Read the model definition and answer for the solid it produces. Units are mm, in the model's axes. Round coordinates to 2 decimals unless told otherwise and drop trailing zeros. Write each loop counter-clockwise with the first axis right and the second up, starting at its lowest first coordinate (ties: lowest second). Pieces come first, ordered by that corner, then holes. Notation, with made-up numbers: (65.25, -26) - (93.25, -26) arc R21 ccw to (93.25, -9) - close; hole circle Ø3 at (-26, 69.25). An arc over 180 degrees is marked (long way). Use one line per item in the form item = value. Start each with the question number.
1) The part is cut by section A-A, the plane y = 3.25. Give the vertices of the cut face in (x, z).
2) The part is cut by section B-B, the plane z = -79.5. Give the vertices of the cut face in (x, y).
3) Consider line 1 along X through (y, z) = (1.05, -15.5); line 2 along Z through (x, y) = (13, 8); line 3 along Z through (x, y) = (57.75, 0.6). Determine where each line is inside the solid, lowest interval first. Write a range as from..to.
4) The part is cut by section D-D, the plane z = -15.5. Give the vertices of the cut face in (x, y).
5) Each of these flat-tipped pins is pushed along its axis until it touches: pin 1 (2 mm diameter, centred on x = 70, y = 3, fed in from -Z); pin 2 (4 mm diameter, centred on x = 111.75, z = -15.5, fed in from +Y); pin 3 (4.5 mm diameter, centred on y = 5, z = -7, fed in from -X). Where does it stop, or does it pass through?
6) The part is cut by section C-C, the plane x = 57.75. Give the vertices of the cut face in (y, z).
from build123d import *

# Parameters (mm, degrees)
SKETCH1_W                = 116
SKETCH1_H                = 100
BOSS_EXTRUDE1_DEPTH      = 1.65
M3_CLEARANCE_HOLE1_D     = 3.2
M3_CLEARANCE_HOLE1_DEPTH = 20
M3_CLEARANCE_HOLE1_TIP   = 0.96137699
SKETCH6_W                = 52.4
SKETCH6_H                = 11.4
SKETCH6_W_2              = 50
SKETCH6_H_2              = 9
EXTRUDE_THIN1_DEPTH      = 9


with BuildPart() as part:
    # Sketch1 → Boss-Extrude1 (new body)
    with BuildSketch(Plane(origin=(0, 0, 0), x_dir=(1, 0, 0), z_dir=(0, 1, 0))):
        with Locations((58, 50)):
            Rectangle(SKETCH1_W, SKETCH1_H)
    extrude(amount=BOSS_EXTRUDE1_DEPTH)

    # M3 Clearance Hole1
    with Locations(Plane(origin=(0, 1.65, 0), x_dir=(1, 0, 0), z_dir=(0, 1, 0))):
        with Locations((4, 15.5), (111.75, 15.5), (57.75, 79.5)):
            Hole(M3_CLEARANCE_HOLE1_D / 2, depth=M3_CLEARANCE_HOLE1_DEPTH)
            with Locations((0, 0, -(M3_CLEARANCE_HOLE1_DEPTH + M3_CLEARANCE_HOLE1_TIP / 2))):  # 118° drill point
                Cone(0, M3_CLEARANCE_HOLE1_D / 2, M3_CLEARANCE_HOLE1_TIP, mode=Mode.SUBTRACT)

    # Sketch6 → Extrude-Thin1 (add)
    with BuildSketch(Plane(origin=(0, 1.65, 0), x_dir=(1, 0, 0), z_dir=(0, 1, 0))):
        with Locations((29, 7.5)):
            Rectangle(SKETCH6_W, SKETCH6_H)
        with Locations((29, 7.5)):
            Rectangle(SKETCH6_W_2, SKETCH6_H_2, mode=Mode.SUBTRACT)
        with Locations((87, 7.5)):
            Rectangle(SKETCH6_W, SKETCH6_H)
        with Locations((87, 7.5)):
            Rectangle(SKETCH6_W_2, SKETCH6_H_2, mode=Mode.SUBTRACT)
    extrude(amount=EXTRUDE_THIN1_DEPTH)


solid = part.part
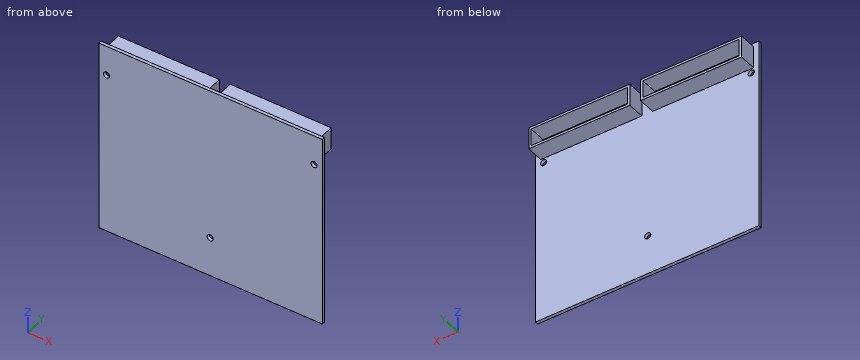
Geometry results:
q1.outline = (2.8, -13.2) - (55.2, -13.2) - (55.2, -1.8) - (2.8, -1.8) - close; (60.8, -13.2) - (113.2, -13.2) - (113.2, -1.8) - (60.8, -1.8) - close; hole (4, -12) - (54, -12) - (54, -3) - (4, -3) - close; hole (62, -12) - (112, -12) - (112, -3) - (62, -3) - close
q2.outline = (0, 0) - (56.15, 0) - (56.15, 1.65) - (0, 1.65) - close; (59.35, 0) - (116, 0) - (116, 1.65) - (59.35, 1.65) - close
q3.line_1 = 0..2.4, 5.6..110.15, 113.35..116
q3.line_2 = -13.2..-12, -3..-1.8
q3.line_3 = -100..-81.1, -77.9..0
q4.outline = (0, 0) - (2.4, 0) - (2.4, 1.65) - (0, 1.65) - close; (5.6, 0) - (110.15, 0) - (110.15, 1.65) - (5.6, 1.65) - close; (113.35, 0) - (116, 0) - (116, 1.65) - (113.35, 1.65) - close
q5.pin_1 = -13.2
q5.pin_2 = 1.65
q5.pin_3 = 2.8
q6.outline = (0, -100) - (1.65, -100) - (1.65, -81.1) - (0, -81.1) - close; (0, -77.9) - (1.65, -77.9) - (1.65, 0) - (0, 0) - close
